from build123d import *

# Parameters (mm, degrees)
F0_W     = 117.475
F0_H     = 117.475
F1_DEPTH = 120.65
F2_T     = -4.7625
F4_D     = 9.525
F6_DEPTH = 0.79375
F9_DEPTH = 117.475


with BuildPart() as f1:
    # F0 (on Top) → F1 (new body)
    with BuildSketch(Plane.XY):
        Rectangle(F0_W, F0_H)
    extrude(amount=F1_DEPTH)

    # F2
    f2_openings = [f1.faces().sort_by_distance(p)[0] for p in [
        (0, 0, 120.65),
    ]]
    offset(amount=F2_T, openings=f2_openings)

    # F4 (through all)
    with Locations(Plane.YZ.offset(58.7375)):
        with Locations((0, 88.9)):
            Hole(F4_D / 2)


with BuildPart() as f6:
    # F5 (on face) → F6 (new body)
    with BuildSketch(Plane(origin=(0, -53.975, 0), x_dir=(-1, 0, 0), z_dir=(0, 1, 0))):
        with BuildLine():
            Line((0, 117.475), (-6.35, 117.475))
            ThreePointArc((-6.35, 117.475), (-8.595064, 116.545064), (-9.525, 114.3))
            Line((-9.525, 114.3), (-9.525, 101.6))
            ThreePointArc((-9.525, 101.6), (-8.595064, 99.354936), (-6.35, 98.425))
            Line((-6.35, 98.425), (6.35, 98.425))
            ThreePointArc((6.35, 98.425), (8.595064, 99.354936), (9.525, 101.6))
            Line((9.525, 101.6), (9.525, 114.3))
            ThreePointArc((9.525, 114.3), (8.595064, 116.545064), (6.35, 117.475))
            Line((6.35, 117.475), (0, 117.475))
        make_face()
        with BuildLine():
            Line((-6.35, 116.68125), (0, 116.68125))
            Line((0, 116.68125), (6.35, 116.68125))
            ThreePointArc((6.35, 116.68125), (8.033798, 115.983798), (8.73125, 114.3))
            Line((8.73125, 114.3), (8.73125, 101.6))
            ThreePointArc((8.73125, 101.6), (8.033798, 99.916202), (6.35, 99.21875))
            Line((6.35, 99.21875), (-6.35, 99.21875))
            ThreePointArc((-6.35, 99.21875), (-8.033798, 99.916202), (-8.73125, 101.6))
            Line((-8.73125, 101.6), (-8.73125, 114.3))
            ThreePointArc((-8.73125, 114.3), (-8.033798, 115.983798), (-6.35, 116.68125))
        make_face(mode=Mode.SUBTRACT)
    extrude(amount=-F6_DEPTH)


with BuildPart() as f1_1:
    add(f1.part)

    # F7: cut F6
    add(f6.part, mode=Mode.SUBTRACT)


with BuildPart() as f9:
    # F8 (on face) → F9 (new body, through all)
    with BuildSketch(Plane.YZ.offset(58.7375)):
        with BuildLine():
            ThreePointArc((0, 93.6625), (4.7625, 88.9), (0, 84.1375))
            Line((0, 84.1375), (19.05, 84.1375))
            ThreePointArc((19.05, 84.1375), (25.785192, 86.927308), (28.575, 93.6625))
            Line((28.575, 93.6625), (28.575, 120.65))
            Line((28.575, 120.65), (19.05, 120.65))
            Line((19.05, 120.65), (19.05, 93.6625))
            Line((19.05, 93.6625), (0, 93.6625))
        make_face()
    extrude(amount=-F9_DEPTH)


with BuildPart() as f1_2:
    add(f1_1.part)

    # F10: cut F9
    add(f9.part, mode=Mode.SUBTRACT)


solid = f1_2.part
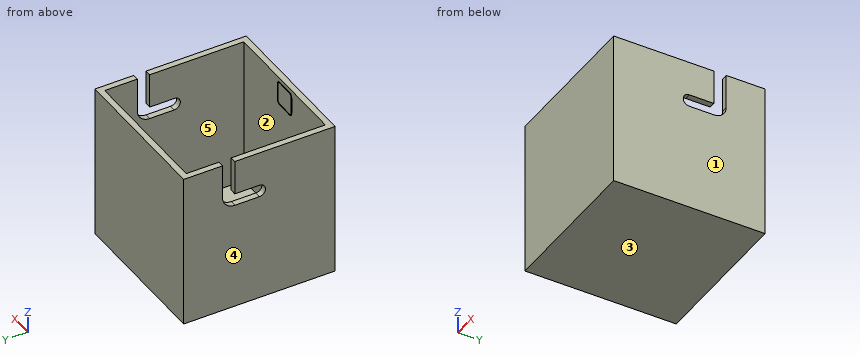
Could you check a few things on this model? Use its own coordinates, in mm. Face numbers are marked on the shaded views. A direction names the side the tool comes from. Coordinates: 2 decimals unless noted, no trailing zeros. Write each loop counter-clockwise with the first axis right and the second up, starting at its lowest first coordinate (ties: lowest second). Pieces come first, ordered by that corner, then holes. Notation, with made-up numbers: M 84,72.25 L 94,72.25 A20 cw 94,83.25 Z; hole C -15,-20.5 d9. An arc over 180 degrees is marked long. One line per question, with ' | ' between items.
1) If we mould it in two halves opening along X, with no side actions, what happens to the marked faces 3, 4 and 5? For each: released by +X, released by -X, zero draft, split by the parting line, or undercut.
Checks:
face 3: zero draft | face 4: released by -X | face 5: undercut
2) For pin 1 Ø6 at (x, y) = (-4.5, 20.5) entering from +Z, with a flat end and sliding along its axis, tell me the tip position at first contact or that it passes through.
Checks:
pin 1: z = 4.76
3) Imagine slicing it at B-B, the plane z = 43. Write out the boundary of the cut face in (x, y) (1 decimal), and give its area (3 significant figures).
Checks:
outline: M -58.7,-58.7 L 58.7,-58.7 L 58.7,58.7 L -58.7,58.7 Z; hole M -54,-54 L 54,-54 L 54,54 L -54,54 Z | area: 2,150 mm²
4) I need wall thicknesses on probe 1 along Y at (x, z) = (17, 81.5) (1 decimal); probe 2 along Z at (x, y) = (-27.5, 7.5). Which ranges of each line are inside material? Lowest first, please. Write a range as [from, to].
Checks:
probe 1: [-58.7, -54], [54, 58.7] | probe 2: [0, 4.76]
5) For the marked faces 1 and 2, which set-ups out of +Z, -Z, +X, -X, +Y, -Y let a thin tool reach every point of the face, with its end or its side?
Checks:
face 1: +Z, -Z, +X, +Y, -Y | face 2: +Z
